CAD build for the part. Positions are in the model's coordinates, mm. A direction names the side the tool comes from. Give positions to 0.01 mm unless a question says otherwise; leave off trailing zeros. Write each loop counter-clockwise with the first axis right and the second up, starting at its lowest first coordinate (ties: lowest second). Pieces come first, ordered by that corner, then holes. Notation, with made-up numbers: (23, 36.5) -> (69, 36.5) arc R16 cw to (69, 46.5) -> close; hole circle Ø7 at (69, 36.5). An arc over 180 degrees is marked (long way). Answer as a JSON object with one key per item and string values.
```python
from build123d import *

# Parameters (mm, degrees)
FILLET1_R = 0.79375


with BuildPart() as part:
    # Sketch1 → Revolve1 (revolve)
    with BuildSketch(Plane(origin=(0, 0, 0), x_dir=(0, 0, -1), z_dir=(1, 0, 0))):
        Polygon((0, 4.7625), (25.4, 4.7625), (25.4, -4.7625), (22.225, -4.7625), (22.225, 1.5875), (0, 1.5875), align=None)
    revolve(axis=Axis((0, -32.325211936, 0), (0, 1, 0)))

    # Fillet1
    fillet1_edges = [part.edges().sort_by_distance(p)[0] for p in [
        (0, 1.5875, 22.225),
        (0, -4.7625, 22.225),
        (0, 4.7625, 25.4),
    ]]
    fillet(fillet1_edges, radius=FILLET1_R)


solid = part.part
```
1) Mould opens along Y. For faces 1 (the flat face through (0, 4.763, 0)), 2 (the flat face through (0, 1.587, 0)), 3 (the cylindrical face through (24.796, -0.458, 5.506)) say: released by +Y, released by -Y, zero draft, split by the parting line, or undercut.
Model answer:
{"face 1": "released by +Y", "face 2": "released by -Y", "face 3": "zero draft"}
2) Slice it at B-B (z = 0). List the corners of the cut face in (x, y) (1 decimal), then the cut area to 3 significant figures.
Model answer:
{"outline": "(-25.4, -4.8) -> (-23, -4.8) arc R0.8 ccw to (-22.2, -4) -> (-22.2, 0.8) arc R0.8 cw to (-21.4, 1.6) -> (21.4, 1.6) arc R0.8 cw to (22.2, 0.8) -> (22.2, -4) arc R0.8 ccw to (23, -4.8) -> (25.4, -4.8) -> (25.4, 4) arc R0.8 ccw to (24.6, 4.8) -> (-24.6, 4.8) arc R0.8 ccw to (-25.4, 4) -> close", "area": "201 mm2"}
3) Wall check: probe 1 along X at (y, z) = (-2.75, 0) (3 decimals); probe 2 along Y at (x, z) = (-12.5, -13.5). Give the ranges that are in metal, low to high.
Model answer:
{"probe 1": "x = -25.4 to -22.225, 22.225 to 25.4", "probe 2": "y = 1.59 to 4.76"}
4) 3-axis set-ups, long thin cutter, end or side, ignore diameter. For faces 4 (the flat face through (-4, -4.762, 23)), 5 (the cylindrical face through (-6.676, -1.554, -21.199)): which of +Z, -Z, +X, -X, +Y, -Y reach the whole face in a straight line?
Model answer:
{"face 4": "+Z, -Z, +X, -X, -Y", "face 5": "-Y"}
5) Slice it at A-A (x = 0). List the corners of the cut face in (y, z) (1 decimal), then the cut area to 3 significant figures.
Model answer:
{"outline": "(-4.8, -25.4) -> (4, -25.4) arc R0.8 ccw to (4.8, -24.6) -> (4.8, 24.6) arc R0.8 ccw to (4, 25.4) -> (-4.8, 25.4) -> (-4.8, 23) arc R0.8 ccw to (-4, 22.2) -> (0.8, 22.2) arc R0.8 cw to (1.6, 21.4) -> (1.6, -21.4) arc R0.8 cw to (0.8, -22.2) -> (-4, -22.2) arc R0.8 ccw to (-4.8, -23) -> close", "area": "201 mm2"}
6) Pin check, flat tips, straight feed: pin 1 (1.5 mm diameter, centred on y = 0, z = -18.5, fed in from +X); pin 2 (2 mm diameter, centred on y = -3, z = -7.5, fed in from -X); pin 3 (1.5 mm diameter, centred on x = 3, y = 4, fed in from +Z). Stop position of each tip, or through.
Model answer:
{"pin 1": "stops at x = 18.17", "pin 2": "stops at x = -24.55", "pin 3": "stops at z = 25.3"}
